```python
from build123d import *

# Parameters (mm, degrees)
SKETCH2_W           = 17.5
SKETCH2_H           = 36
SKETCH3_R           = 2.5
BOSS_EXTRUDE1_DEPTH = 16.5
SKETCH4_R           = 1.5
SKETCH4_R_2         = 4
CUT_EXTRUDE2_DEPTH  = 5


with BuildPart() as part:
    # Sketch2 → Revolve1 (revolve)
    with BuildSketch(Plane.XY, mode=Mode.PRIVATE) as revolve1_sk:
        with Locations((8.75, 0)):
            Rectangle(SKETCH2_W, SKETCH2_H)
    revolve(revolve1_sk.sketch.rotate(Axis((0, 18, 0), (0, -1, 0)), 180), axis=Axis((0, 18, 0), (0, -1, 0)))

    # Sketch3 → Boss-Extrude1 (add)
    with BuildSketch(Plane(origin=(0, 18, 0), x_dir=(1, 0, 0), z_dir=(0, 1, 0))):
        Circle(SKETCH3_R)
    extrude(amount=BOSS_EXTRUDE1_DEPTH)

    # Sketch4 → Cut-Extrude2 (cut)
    with BuildSketch(Plane.XZ.offset(18)):
        with Locations((0, 9.5)):
            Circle(SKETCH4_R)
        with Locations((0, -9.5)):
            Circle(SKETCH4_R)
        with Locations((12.5, 0)):
            Circle(SKETCH4_R)
        with Locations((-12.5, 0)):
            Circle(SKETCH4_R)
        with Locations((-8.838834765, 8.838834765)):
            Circle(SKETCH4_R_2)
        with Locations((8.838834765, -8.838834765)):
            Circle(SKETCH4_R_2)
        with Locations((-8.838834765, -8.838834765)):
            Circle(SKETCH4_R_2)
        with Locations((8.838834765, 8.838834765)):
            Circle(SKETCH4_R_2)
    extrude(amount=-CUT_EXTRUDE2_DEPTH, mode=Mode.SUBTRACT)


solid = part.part
```
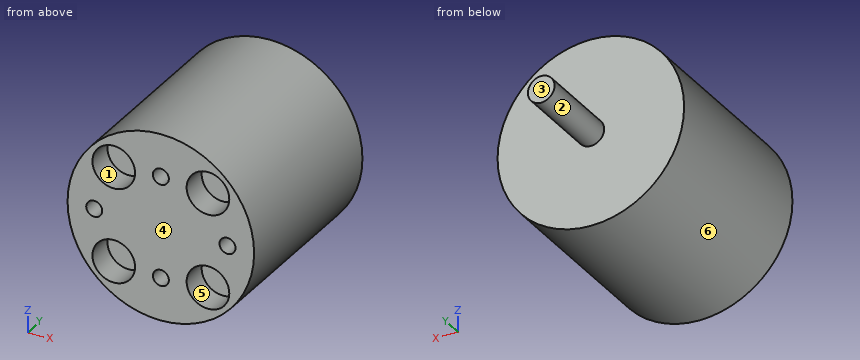
Check sheet for the modelled part. Datum: model origin and axes. Units: mm. Face numbers are marked on the shaded views. A direction names the side the tool comes from. Coordinates: 2 decimals unless noted, no trailing zeros. Write each loop counter-clockwise with the first axis right and the second up, starting at its lowest first coordinate (ties: lowest second). Pieces come first, ordered by that corner, then holes. Notation, with made-up numbers: (-34.75, 18.25) -> (-21.75, 18.25) arc R12 cw to (-21.75, 22.25) -> close; hole circle Ø9 at (28, 11). An arc over 180 degrees is marked (long way). Use a Markdown table: item, result.
1. Tool access check on the marked faces 1, 2 and 3. Record the directions out of +Z, -Z, +X, -X, +Y, -Y that give a thin tool (end or side, any length) a straight path to the whole face; none if there is none.
Reported:
| item | result |
|---|---|
| face 1 | -Y |
| face 2 | +Y |
| face 3 | +Z, -Z, +X, -X, +Y |
2. Sectioned sample at B-B (x = 0). Enter the section's corners in (y, z).
Reported:
| item | result |
|---|---|
| outline | (-18, -17.5) -> (18, -17.5) -> (18, -2.5) -> (34.5, -2.5) -> (34.5, 2.5) -> (18, 2.5) -> (18, 17.5) -> (-18, 17.5) -> (-18, 11) -> (-13, 11) -> (-13, 8) -> (-18, 8) -> (-18, -8) -> (-13, -8) -> (-13, -11) -> (-18, -11) -> close |
3. Scan lines: line 1 along Y through (x, z) = (-11, 11.5); line 2 along Y through (x, z) = (-7.5, -15); line 3 along Z through (x, y) = (8.5, -15). Record each from-to range of solid material in increasing order.
Reported:
| item | result |
|---|---|
| line 1 | y = -13 to 18 |
| line 2 | y = -18 to 18 |
| line 3 | z = -15.3 to -12.82, -4.85 to 4.85, 12.82 to 15.3 |
4. Sectioned sample at A-A (z = 0). Enter the section's corners in (x, y), plus the area to 3 significant figures.
Reported:
| item | result |
|---|---|
| outline | (-17.5, -18) -> (-14, -18) -> (-14, -13) -> (-11, -13) -> (-11, -18) -> (11, -18) -> (11, -13) -> (14, -13) -> (14, -18) -> (17.5, -18) -> (17.5, 18) -> (2.5, 18) -> (2.5, 34.5) -> (-2.5, 34.5) -> (-2.5, 18) -> (-17.5, 18) -> close |
| area | 1,310 mm2 |
5. Sectioned sample at D-D (y = 10.5). Enter the section's corners in (x, z), plus the area to 3 significant figures.
Reported:
| item | result |
|---|---|
| outline | circle Ø35 at (0, 0) |
| area | 962 mm2 |
6. Sectioned sample at C-C (y = -14.5). Give the number of separate pieces and of enclosed holes in the cut face, plus the area to 3 significant figures.
Reported:
| item | result |
|---|---|
| separate pieces | 1 |
| enclosed holes | 8 |
| area | 733 mm2 |
7. Go/stop test with flat-tipped pins: pin 1 Ø10 at (x, y) = (10, 16) entering from -Z; pin 2 Ø6.5 at (x, z) = (8.84, -8.84) entering from +Y; pin 3 Ø5 at (x, z) = (8, 9) entering from -Y; pin 4 Ø10 at (y, z) = (27.5, -9) entering from -X. Record where each tip stops, or that it passes through.
Reported:
| item | result |
|---|---|
| pin 1 | stops at z = -16.77 |
| pin 2 | stops at y = 18 |
| pin 3 | stops at y = -13 |
| pin 4 | passes through |
8. Release check for a two-part mould opening along X. For the marked faces 4, 5 and 6 record: pulls with the +X half, pulls with the -X half, needs draft (parallel to the pull), parting line crosses it, or undercut.
Reported:
| item | result |
|---|---|
| face 4 | needs draft |
| face 5 | undercut |
| face 6 | parting line crosses it |
